Geometry check sheet. Reference: drawing and pictorial views, mm from the part's lowest x, y, z. A direction names the side the tool comes from. Coordinates: 2 decimals unless noted, no trailing zeros. Loops run counter-clockwise (first coordinate to the right, second up) from the corner with the lowest first, then second, coordinate; pieces in that order, holes last. Notation, with made-up numbers: (17.5, 72.5) -> (39.5, 72.5) arc R9 ccw to (39.5, 83.5) -> close; hole circle Ø4 at (-27, -1). An arc over 180 degrees is marked (long way). Use one line per item in the form item = value.
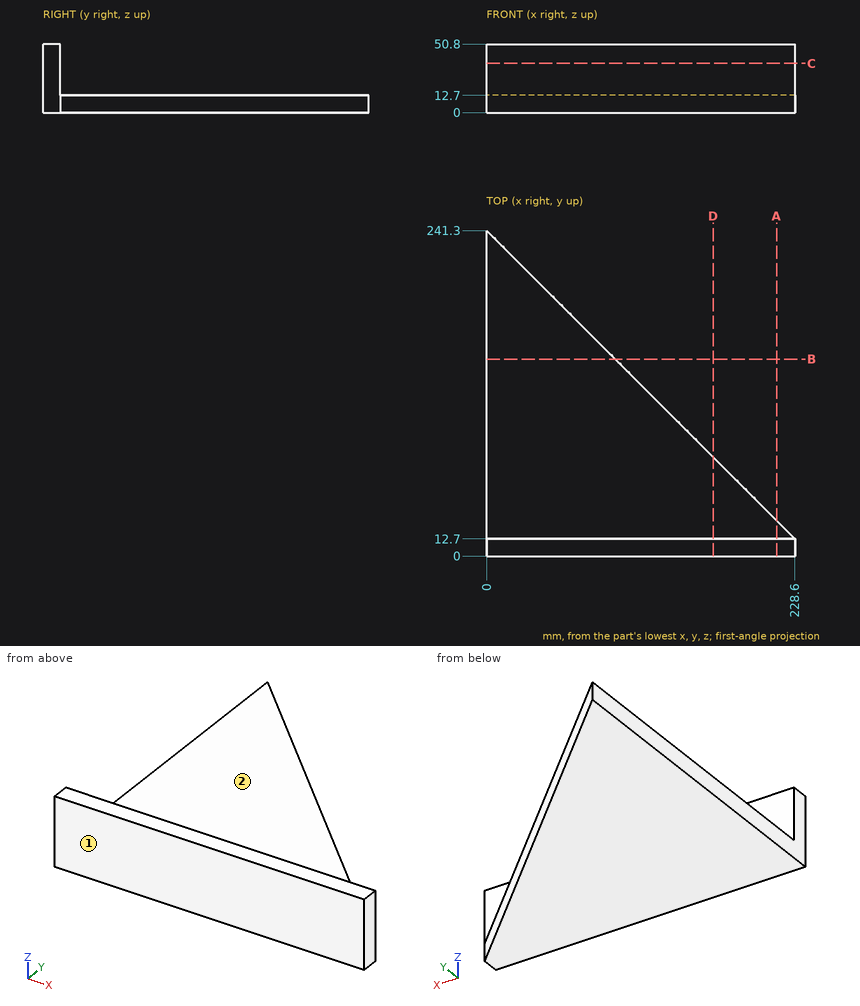
(1) Section check B-B, the plane y = 146. Record the boundary of the cut face in (x, z), plus the area to 3 significant figures.
Established:
outline = (0, 0) -> (95.3, 0) -> (95.3, 12.7) -> (0, 12.7) -> close
area = 1,210 mm²
(2) Section check D-D, the plane x = 168. Record the boundary of the cut face in (y, z).
Established:
outline = (0, 0) -> (73.3, 0) -> (73.3, 12.7) -> (12.7, 12.7) -> (12.7, 50.8) -> (0, 50.8) -> close
(3) Section check A-A, the plane x = 215. Record the boundary of the cut face in (y, z).
Established:
outline = (0, 0) -> (26.3, 0) -> (26.3, 12.7) -> (12.7, 12.7) -> (12.7, 50.8) -> (0, 50.8) -> close
(4) Scan lines: line 1 along Y through (x, z) = (184, 30); line 2 along Y through (x, z) = (214, 8.5). Record each from-to range of solid material in increasing order.
Established:
line_1 = 0 to 12.7
line_2 = 0 to 27.3
(5) Tool access check on the marked faces 1 and 2. Record the directions out of +Z, -Z, +X, -X, +Y, -Y that give a thin tool (end or side, any length) a straight path to the whole face; none if there is none.
Established:
face_1 = +Z, -Z, +X, -X, -Y
face_2 = +Z, +X, -X, +Y
(6) Go/stop test with flat-tipped pins: P1, Ø12, axis at x = 61, z = 8.5, coming from the -Y side; P2, Ø10, axis at x = 67, z = 16.5, coming from the +Y side; P3, Ø1, axis at x = 96, z = 33.5, coming from the +Y side. Record where each tip stops, or that it passes through.
Established:
P1 = 0
P2 = 177.55
P3 = 12.7
(7) Section check C-C, the plane z = 36.5. Record the boundary of the cut face in (x, y).
Established:
outline = (0, 0) -> (228.6, 0) -> (228.6, 12.7) -> (0, 12.7) -> close
